Can you work these out from the model? Positions are in its coordinate system, mm. Face numbers are marked on the shaded views. Give positions to 0.01 mm unless a question says otherwise; leave off trailing zeros. Loops run counter-clockwise (first coordinate to the right, second up) from the corner with the lowest first, then second, coordinate; pieces in that order, holes last. Notation, with made-up numbers: M -37.75,18 L 7.25,18 A26 ccw 7.25,42 Z; hole C -11.5,82.25 d3. An arc over 180 degrees is marked long. Put each result on its own line as item: value. Start each with the question number.
1) Please list where these lines run through material, in increasing order: line 1 along Z through (x, y) = (0, -42.75); line 2 along Z through (x, y) = (17, -41). Write a range as from..to.
2) If we mould it in two halves opening along Z, with no side actions, what happens to the marked faces 1, 2 and 3? For each: +Z half, -Z half, draft (parallel to the pull), parting line (faces both ways), or undercut.
3) Imagine slicing it at B-B (z = 31). Write out the boundary of the cut face in (x, y), then the cut area to 3 significant figures.
4) Imagine slicing it at A-A (x = 0). Write out the boundary of the cut face in (y, z).
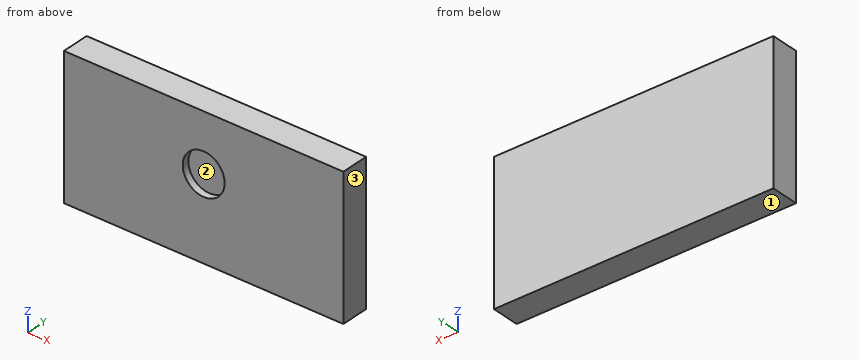
from build123d import *

# Parameters (mm, degrees)
F0_W     = 508
F0_H     = 254
F1_DEPTH = 50.8
F2_R     = 38.1
F3_DEPTH = 12.7
F4_R     = 25.4
F5_DEPTH = 12.7
F6_R     = 50.631334
F7_DEPTH = 25.4


with BuildPart() as f1:
    # F0 (on Front) → F1 (new body)
    with BuildSketch(Plane.XZ):
        Rectangle(F0_W, F0_H)
    extrude(amount=F1_DEPTH)

    # F2 (on face) → F3 (cut)
    with BuildSketch(Plane.XZ.offset(50.8)):
        with Locations((0, 22.220068)):
            Circle(F2_R)
    extrude(amount=-F3_DEPTH, mode=Mode.SUBTRACT)

    # F4 (on face) → F5 (join)
    with BuildSketch(Plane.XZ.offset(50.8)):
        with Locations((-48.272954, -19.034895)):
            Circle(F4_R)
    extrude(amount=-F5_DEPTH)

    # F6 (on face) → F7 (join)
    with BuildSketch(Plane.XZ.offset(50.8)):
        with Locations((-68.167724, -34.581438)):
            Circle(F6_R)
    extrude(amount=-F7_DEPTH)


solid = f1.part
Recorded:
1. line 1: -127..-15.88, 60.32..127
1. line 2: -127..-11.88, 56.32..127
2. face 1: -Z half
2. face 2: undercut
2. face 3: draft
3. outline: M -254,-50.8 L -37.07,-50.8 L -37.07,-38.1 L 37.07,-38.1 L 37.07,-50.8 L 254,-50.8 L 254,0 L -254,0 Z
3. area: 24,900 mm²
4. outline: M -50.8,-127 L 0,-127 L 0,127 L -50.8,127 L -50.8,60.32 L -38.1,60.32 L -38.1,-15.88 L -50.8,-15.88 Z
